Geometry check sheet. Reference: drawing and pictorial views, mm from the part's lowest x, y, z. A direction names the side the tool comes from. Round coordinates to 2 decimals unless told otherwise and drop trailing zeros. Write each loop counter-clockwise with the first axis right and the second up, starting at its lowest first coordinate (ties: lowest second). Pieces come first, ordered by that corner, then holes. Notation, with made-up numbers: M 52.25,-24.75 L 79.25,-24.75 A15 ccw 79.25,-1.75 Z; hole C 50.5,40 d3. An arc over 180 degrees is marked long. Answer in a Markdown table with one row per item.
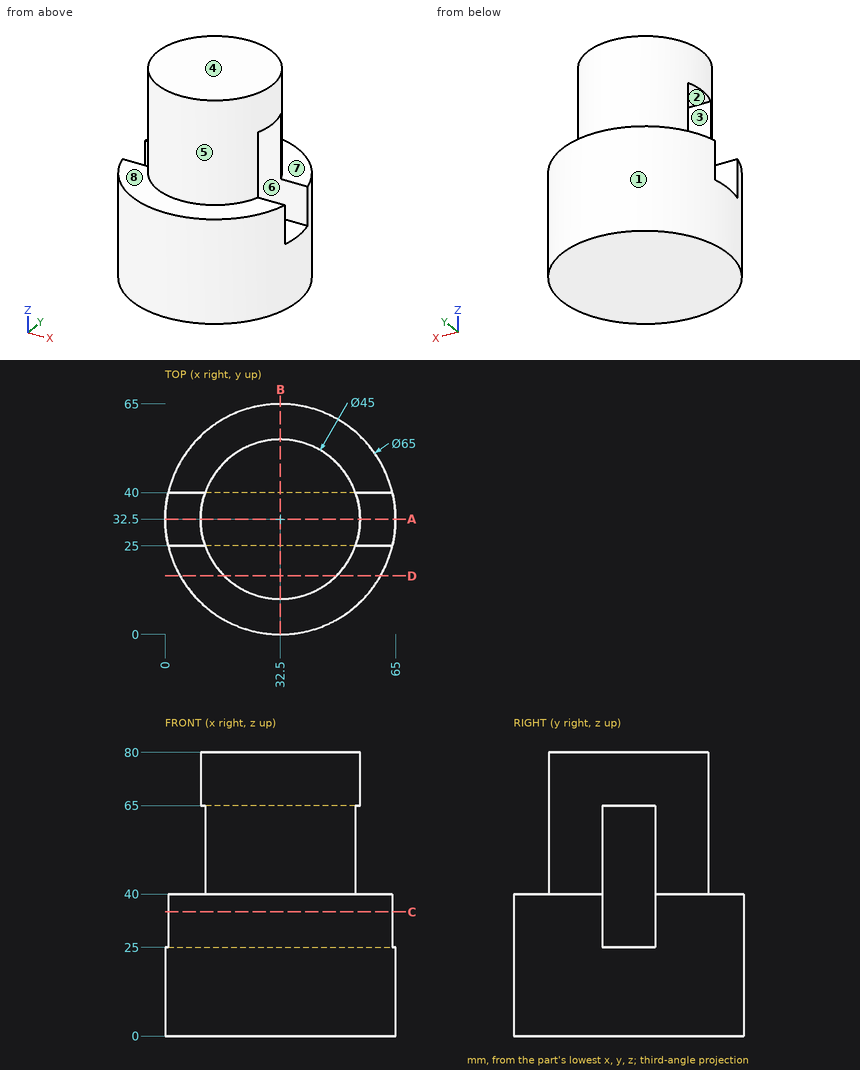
1. Section check D-D, the plane y = 16.5. Record the cut outline in (x, z), and give its area (3 significant figures).
Found:
| item | result |
|---|---|
| outline | M 4.21,0 L 60.79,0 L 60.79,40 L 48.32,40 L 48.32,80 L 16.68,80 L 16.68,40 L 4.21,40 Z |
| area | 3,530 mm2 |
2. Section check C-C, the plane z = 35. Record the cut outline in (x, y), and give its area (3 significant figures).
Found:
| item | result |
|---|---|
| outline | M 0.88,25 A32.5 ccw 64.12,25 Z; M 0.88,40 L 64.12,40 A32.5 ccw Z |
| area | 2,350 mm2 |
3. Draft check along Y on the marked faces 1, 2, 3 and 4. Enter one of: +Y half, -Y half, draft (parallel to the pull), parting line (faces both ways), or undercut.
Found:
| item | result |
|---|---|
| face 1 | parting line |
| face 2 | undercut |
| face 3 | undercut |
| face 4 | draft |
4. Go/stop test with flat-tipped pins: pin 1 (8 mm diameter, centred on x = 44.5, z = 45, fed in from -Y); pin 2 (1 mm diameter, centred on y = 12, z = 45, fed in from -X); pin 3 (10 mm diameter, centred on y = 27.5, z = 71.5, fed in from -X). Record where each tip stops, or that it passes through.
Found:
| item | result |
|---|---|
| pin 1 | stops at y = 11.47 |
| pin 2 | stops at x = 22.19 |
| pin 3 | stops at x = 10 |
5. Section check A-A, the plane y = 32.5. Record the cut outline in (x, z), and give its area (3 significant figures).
Found:
| item | result |
|---|---|
| outline | M 0,0 L 65,0 L 65,25 L 0,25 Z; M 10,65 L 55,65 L 55,80 L 10,80 Z |
| area | 2,300 mm2 |
6. Access from +Z, -Z, +X, -X, +Y, -Y to the whole of each face (thin tool, end or side, straight path). Record for the marked faces 5, 6, 7 and 8.
Found:
| item | result |
|---|---|
| face 5 | +Z |
| face 6 | +X, -X |
| face 7 | +Z, +Y |
| face 8 | +Z, -Y |
7. Scan lines: L1, parallel to Z at x = 24, y = 29; L2, parallel to Z at x = 46, y = 11.5; L3, parallel to Z at x = 8.5, y = 33.5. Record each from-to range of solid material in increasing order.
Found:
| item | result |
|---|---|
| L1 | z = 0 to 25, 65 to 80 |
| L2 | z = 0 to 40 |
| L3 | z = 0 to 25 |
8. Section check B-B, the plane x = 32.5. Record the cut outline in (y, z).
Found:
| item | result |
|---|---|
| outline | M 0,0 L 65,0 L 65,40 L 55,40 L 55,80 L 10,80 L 10,40 L 0,40 Z; hole M 25,25 L 40,25 L 40,65 L 25,65 Z |
